Design review of the part built by this model. Coordinates are the model's own, in mm. A direction names the side the tool comes from. Give positions to 0.01 mm unless a question says otherwise; leave off trailing zeros. Order: outer loops, then holes, each group sorted by start corner. A loop starts at its lowest first (then second) coordinate and runs counter-clockwise, first axis right, second up. Notation, with made-up numbers: (11.25, 67.5) -> (23.25, 67.5) arc R23 cw to (23.25, 81.5) -> close; hole circle Ø4 at (-1.5, 67.5). An arc over 180 degrees is marked (long way). Answer in a Markdown table with one row per item. Add a question column.
```python
from build123d import *

# Parameters (mm, degrees)
SKETCH1_R             = 3.175
BOSS_EXTRUDE1_DEPTH   = 4.7625
BOSS_EXTRUDE1_2_DEPTH = 4.7625
BOSS_EXTRUDE1_3_DEPTH = 4.7625
BOSS_EXTRUDE1_4_DEPTH = 4.7625
BOSS_EXTRUDE1_5_DEPTH = 4.7625
SKETCH2_R             = 1.984375
BOSS_EXTRUDE2_DEPTH   = 9.525
BOSS_EXTRUDE3_DEPTH   = 3.175
SKETCH5_R             = 2
CUT_EXTRUDE1_DEPTH    = 207.765399971
CUT_EXTRUDE2_DEPTH    = 0.5
CHAMFER1_SIZE         = 7.62
CHAMFER1_SIZE_2       = 9.081162376


with BuildPart() as part:
    # Sketch1 → Boss-Extrude1 (new body)
    with BuildSketch(Plane.XY):
        with Locations(Location((-78.19292114, 62.356773808, 0), (0, 0, 180))):
            Circle(SKETCH1_R)
    extrude(amount=BOSS_EXTRUDE1_DEPTH)



with BuildPart() as body_2:
    # Sketch1 → Boss-Extrude1 2 (new body)
    with BuildSketch(Plane.XY):
        with Locations(Location((-97.504977817, -22.254874907, 0), (0, 0, 180))):
            Circle(SKETCH1_R)
    extrude(amount=BOSS_EXTRUDE1_2_DEPTH)


with BuildPart() as body_3:
    # Sketch1 → Boss-Extrude1 3 (new body)
    with BuildSketch(Plane.XY):
        with Locations(Location((-43.393797458, -90.108148901, 0), (0, 0, 180))):
            Circle(SKETCH1_R)
    extrude(amount=BOSS_EXTRUDE1_3_DEPTH)


with BuildPart() as body_4:
    # Sketch1 → Boss-Extrude1 4 (new body)
    with BuildSketch(Plane.XY):
        with BuildLine():
            Line((-88.191845565, 53.571060584), (-82.764655069, 50.274379933))
            ThreePointArc((-82.764655069, 50.274379933), (-94.409581696, 21.548370942), (-96.381613527, -9.385413164))
            Line((-96.381613527, -9.385413164), (-102.701719332, -10.000850093))
            ThreePointArc((-102.701719332, -10.000850093), (-100.600373938, 22.961378873), (-88.191845565, 53.571060584))
        make_face()
    extrude(amount=BOSS_EXTRUDE1_4_DEPTH)


with BuildPart() as body_5:
    # Sketch1 → Boss-Extrude1 5 (new body)
    with BuildSketch(Plane.XY):
        with BuildLine():
            Line((-90.909011383, -33.362449786), (-96.870258031, -35.550151411))
            ThreePointArc((-96.870258031, -35.550151411), (-80.675236097, -64.336353929), (-56.214495182, -86.53086552))
            Line((-56.214495182, -86.53086552), (-52.755141633, -81.20588918))
            ThreePointArc((-52.755141633, -81.20588918), (-75.710606183, -60.377193687), (-90.909011383, -33.362449786))
        make_face()
    extrude(amount=BOSS_EXTRUDE1_5_DEPTH)


with BuildPart() as part_1:
    add(part.part)

    add(body_2.part)  # Boss-Extrude2 merges body 2

    add(body_3.part)  # Boss-Extrude2 merges body 3
    # Sketch2 → Boss-Extrude2 (add)
    with BuildSketch(Plane.XY):
        with BuildLine():
            Line((-82.430084054, 80.927094637), (-136.637001873, 66.402394783))
            ThreePointArc((-136.637001873, 66.402394783), (-143.425587422, 61.866406938), (-146.05, 54.13513679))
            Line((-146.05, 54.13513679), (-146.05, -127))
            ThreePointArc((-146.05, -127), (-140.470384182, -140.470384182), (-127, -146.05))
            Line((-127, -146.05), (-51.469574148, -146.05))
            ThreePointArc((-51.469574148, -146.05), (-43.738303999, -143.425587422), (-39.202316154, -136.637001873))
            Line((-39.202316154, -136.637001873), (-29.247808511, -99.486273586))
            ThreePointArc((-29.247808511, -99.486273586), (-30.083781104, -90.666124862), (-36.482937232, -84.53875393))
            ThreePointArc((-36.482937232, -84.53875393), (-89.766487514, -20.488614994), (-69.549981311, 60.337432202))
            ThreePointArc((-69.549981311, 60.337432202), (-68.376222335, 75.395171012), (-82.430084054, 80.927094637))
        make_face()
        with Locations((-136.525, 44.45)):
            Circle(SKETCH2_R, mode=Mode.SUBTRACT)
        with Locations((-136.525, -31.75)):
            Circle(SKETCH2_R, mode=Mode.SUBTRACT)
        with Locations((-136.525, -107.95)):
            Circle(SKETCH2_R, mode=Mode.SUBTRACT)
        with Locations((-57.15, -136.525)):
            Circle(SKETCH2_R, mode=Mode.SUBTRACT)
        with Locations((-107.95, -136.525)):
            Circle(SKETCH2_R, mode=Mode.SUBTRACT)
    extrude(amount=-BOSS_EXTRUDE2_DEPTH)


    add(body_4.part)  # Boss-Extrude3 merges body 4

    add(body_5.part)  # Boss-Extrude3 merges body 5
    # Sketch3 → Boss-Extrude3 (add)
    with BuildSketch(Plane.XY.offset(4.7625)):
        with BuildLine():
            Line((-81.407857445, 49.45020977), (-88.191845565, 53.571060584))
            ThreePointArc((-88.191845565, 53.571060584), (-100.600373938, 22.961378873), (-102.701719332, -10.000850093))
            Line((-102.701719332, -10.000850093), (-94.801587075, -9.231553932))
            ThreePointArc((-94.801587075, -9.231553932), (-92.861883635, 21.195118959), (-81.407857445, 49.45020977))
        make_face()
        with BuildLine():
            Line((-96.870258031, -35.550151411), (-89.418699721, -32.815524379))
            ThreePointArc((-89.418699721, -32.815524379), (-74.469448705, -59.387403627), (-51.890303245, -79.874645095))
            Line((-51.890303245, -79.874645095), (-56.214495182, -86.53086552))
            ThreePointArc((-56.214495182, -86.53086552), (-80.675236097, -64.336353929), (-96.870258031, -35.550151411))
        make_face()
    extrude(amount=-BOSS_EXTRUDE3_DEPTH)


with BuildPart() as body_2_2:
    # Mirror2: mirrored copy
    add(part_1.part.mirror(Plane(origin=(0, 0, 0), x_dir=(0, 0, 1), z_dir=(1, 0, 0))))

    # Sketch5 → Cut-Extrude1 (cut, through all)
    with BuildSketch(Plane.XY):
        with Locations((119.458619614, -70.809673068)):
            Circle(SKETCH5_R)
        with Locations((112.387551802, -63.738605256)):
            Circle(SKETCH5_R)
        with Locations((78.163583592, -97.962573466)):
            Circle(SKETCH5_R)
        with Locations((85.234651404, -105.033641277)):
            Circle(SKETCH5_R)
        Polygon((106.023590771, -63.031498475), (77.456476811, -91.598612435), (91.598612435, -105.740748059), (120.165726395, -77.173634099), align=None)
    extrude(amount=-CUT_EXTRUDE1_DEPTH, mode=Mode.SUBTRACT)

    # Sketch6 → Cut-Extrude2 (cut, symmetric)
    with BuildSketch(Plane(origin=(91.598612435, -91.598612435, 0), x_dir=(0, 0, -1), z_dir=(0.7071067811865488, -0.7071067811865462, 0))):
        Polygon((9.525, 30.4), (9.525, 36.9), (7.825, 30.4), align=None)
        Polygon((7.825, -10), (9.525, -10), (9.525, -16.5), align=None)
    extrude(amount=CUT_EXTRUDE2_DEPTH, both=True, mode=Mode.SUBTRACT)

    # Chamfer1
    # the kernel refuses this chamfer: 9.081162376, 7.62 mm, written as the material it takes off along each edge
    with BuildSketch(Plane(origin=(0, 0, -9.525), x_dir=(0.15246082974719, -0.9883095139645264, 0), z_dir=(-0.9883095139645264, -0.15246082974719, 0))) as chamfer1_piece_1:
        Polygon((92.075, CHAMFER1_SIZE), (92.075 + CHAMFER1_SIZE_2, 0), (92.075, 0), align=None)
    revolve(axis=Axis((0, 0, -9.525), (0, 0, 1)), revolution_arc=136.746589735, mode=Mode.SUBTRACT)


solid = body_2_2.part
```
1) Mouldability with a two-part tool opening along Z and no side actions: class faces 6 (the face through (101, -56, -9.525)), 7 (the face through (114.757, -69.147, -9.041)), 8 (the face through (94.312, 21.973, 0.783)), 9 (the face through (93, 23, 1.588)) as +Z half, -Z half, draft (parallel to the pull), parting line (faces both ways), or undercut.
2) For L1, parallel to Z at x = 138.5, y = -106.5 (3 decimals); L2, parallel to Y at x = 101.5, z = -5; L3, parallel to Y at x = 57.15, z = -7, list the stretches that pass through material, from the lowest coordinate up.
3) Machinability: for faces 1 (the face through (143.354, 61.958, -4.696)), 2 (the face through (105.68, -91.66, -4.7)), 3 (the face through (94.333, -22.394, 2.348)), 4 (the face through (74.7, -59.1, 3.2)), 5 (the face through (75.438, -60.717, 0.783)), which of the approach directions +Z, -Z, +X, -X, +Y, -Y give a long, thin tool a straight path to every point of the face, cutting with its end or side? Answer none if there is none.
4) Add section A-A, the plane z = -4. Give the number of separate pieces and of enclosed holes in the cut face, and give its area (3 significant figures).
5) Clearance check with flat-ended pins moving along their axes: P1, Ø5, axis at x = 112.39, y = -63.74, coming from the +Z side; P2, Ø12.5, axis at x = 89, y = 6.5, coming from the -Z side; P3, Ø3, axis at y = 1.5, z = -2.5, coming from the -X side; P4, Ø3.5, axis at x = 136.525, y = -107.95, coming from the -Z side. State where each tip first meets the part, or that it passes through.
6) Add section B-B, the plane y = -118. Write out the cut boundary in (x, z) (3 decimals).
Verdict:
| question | item | result |
|---|---|---|
| 1 | face 6 | -Z half |
| 1 | face 7 | draft |
| 1 | face 8 | undercut |
| 1 | face 9 | undercut |
| 2 | L1 | z = -9.525 to 0 |
| 2 | L2 | y = -146.05 to -95.84, -67.56 to 75.82 |
| 2 | L3 | y = -146.05 to -138.51, -134.54 to -79.79 |
| 3 | face 1 | +Z, -Z, +X, +Y |
| 3 | face 2 | +Z, -Z |
| 3 | face 3 | +Z |
| 3 | face 4 | +Z, -X |
| 3 | face 5 | -X |
| 4 | separate pieces | 1 |
| 4 | enclosed holes | 10 |
| 4 | area | 16,000 mm2 |
| 5 | P1 | stops at z = 0 |
| 5 | P2 | stops at z = -4.77 |
| 5 | P3 | stops at x = 92.03 |
| 5 | P4 | passes through |
| 6 | outline | (34.209, -9.525) -> (146.05, -9.525) -> (146.05, 0) -> (34.209, 0) -> close |
